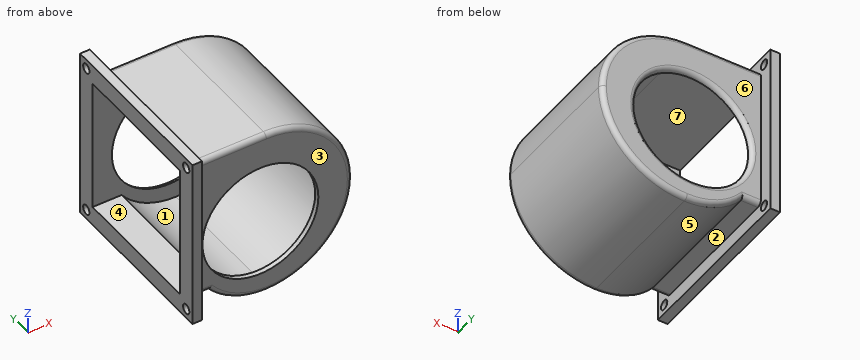
from build123d import *

# Parameters (mm, degrees)
PAD_DEPTH       = 28
THICKNESS_T     = 2
SKETCH001_R     = 24
POCKET_DEPTH    = 60.001
FILLET_R        = 1.9
SKETCH002_W     = 72
SKETCH002_H     = 72
SKETCH002_W_2   = 56
SKETCH002_H_2   = 56
PAD001_DEPTH    = 4
SKETCH003_R     = 2
POCKET001_DEPTH = 5


with BuildPart() as part:
    # Sketch → Pad (new body, symmetric)
    with BuildSketch(Plane.XZ):
        with BuildLine():
            Line((-32, -20), (-32, 36))
            Line((-32, 36), (2.5, 36))
            ThreePointArc((36, 2.5), (26.188077, 26.188077), (2.5, 36))
            ThreePointArc((2.5, -31), (26.188077, -21.188077), (36, 2.5))
            ThreePointArc((-19.994444, -20), (-10.019984, -28.102734), (2.5, -31))
            Line((-32, -20), (-19.994444, -20))
        make_face()
    extrude(amount=PAD_DEPTH, both=True)

    # Thickness
    thickness_openings = [part.faces().sort_by_distance(p)[0] for p in [
        (-32, 0, 8),
    ]]
    offset(amount=THICKNESS_T, openings=thickness_openings)

    # Sketch001 (on Face16 of Thickness) → Pocket (cut, through all)
    with BuildSketch(Plane.XZ.offset(30)):
        Circle(SKETCH001_R)
    extrude(amount=-POCKET_DEPTH, mode=Mode.SUBTRACT)

    # Fillet
    fillet_edges = [part.edges().sort_by_distance(p)[0] for p in [
        (-24, 30, 0),
    ]]
    fillet(fillet_edges, radius=FILLET_R)

    # Sketch002 (on Face3 of Fillet) → Pad001 (join)
    with BuildSketch(Plane(origin=(-32, 0, 0), x_dir=(0, -1, 0), z_dir=(-1, 0, 0))):
        with Locations((0, 8)):
            Rectangle(SKETCH002_W, SKETCH002_H)
        with Locations((0, 8)):
            Rectangle(SKETCH002_W_2, SKETCH002_H_2, mode=Mode.SUBTRACT)
    extrude(amount=-PAD001_DEPTH)

    # Sketch003 (on Face25 of Pad001) → Pocket001 (cut)
    with BuildSketch(Plane(origin=(-32, 0, 0), x_dir=(0, -1, 0), z_dir=(-1, 0, 0))):
        with Locations((-32, 40)):
            Circle(SKETCH003_R)
        with Locations((32, 40)):
            Circle(SKETCH003_R)
        with Locations((32, -24)):
            Circle(SKETCH003_R)
        with Locations((-32, -24)):
            Circle(SKETCH003_R)
    extrude(amount=-POCKET001_DEPTH, mode=Mode.SUBTRACT)


solid = part.part
Here's how the part is built. I have some questions about the finished solid (model axes, mm). Face numbers are marked on the shaded views. A direction names the side the tool comes from. Round coordinates to 2 decimals unless told otherwise and drop trailing zeros. Order: outer loops, then holes, each group sorted by start corner. A loop starts at its lowest first (then second) coordinate and runs counter-clockwise, first axis right, second up. Notation, with made-up numbers: (74.25, 6.25) -> (117.25, 6.25) arc R29 ccw to (117.25, 39.25) -> close; hole circle Ø11 at (73.25, 57.5). An arc over 180 degrees is marked (long way). Use CSV: the item, a comma, the result in double quotes.
1. I want a section at C-C on y = -16.5. List the corners of the cut face in (x, z) for me, and give its area (3 significant figures).
Recorded:
outline,"(-32, -28) -> (-28, -28) -> (-28, -22) -> (-20.95, -22) arc R30.5 ccw to (2.5, -33) arc R35.5 ccw to (38, 2.5) arc R35.5 ccw to (2.5, 38) -> (-28, 38) -> (-28, 44) -> (-32, 44) -> (-32, 36) -> (2.5, 36) arc R33.5 cw to (36, 2.5) arc R33.5 cw to (2.5, -31) arc R28.5 cw to (-19.99, -20) -> (-32, -20) -> close"
area,"409 mm2"
2. I need wall thicknesses on line 1 along Z through (x, y) = (-29.35, -32); line 2 along Z through (x, y) = (-26, -3); line 3 along X through (y, z) = (14.5, -24.5). Which ranges of each line are inside material? Lowest first, please.
Recorded:
line 1,"z = -28 to -26, -22 to 38, 42 to 44"
line 2,"z = -22 to -20, 36 to 38"
line 3,"x = -32 to -28, -18.62 to -15.62, 22.33 to 25.55"
3. I want a section at A-A on y = -32. List the corners of the cut face in (x, z) for me.
Recorded:
outline,"(-32, -28) -> (-28, -28) -> (-28, -26) -> (-32, -26) -> close; (-32, -22) -> (-28, -22) -> (-28, 38) -> (-32, 38) -> close; (-32, 42) -> (-28, 42) -> (-28, 44) -> (-32, 44) -> close"
4. I want a section at B-B on z = 40. List the corners of the cut face in (x, y) for me.
Recorded:
outline,"(-32, -36) -> (-28, -36) -> (-28, -34) -> (-32, -34) -> close; (-32, -30) -> (-28, -30) -> (-28, 30) -> (-32, 30) -> close; (-32, 34) -> (-28, 34) -> (-28, 36) -> (-32, 36) -> close"
5. I'm going to push flat-ended pins straight in: P1, Ø10, axis at x = -22.5, y = 20.5, coming from the -Z side; P2, Ø12, axis at y = 27.5, z = -17, coming from the -X side; P3, Ø3.5, axis at x = -25.5, y = 12.5, coming from the -Z side; P4, Ø5, axis at x = -0.5, z = 22, coming from the +Y side. Where does each tip first touch, or does it pass through?
Recorded:
P1,"stops at z = -25.53"
P2,"stops at x = -32"
P3,"stops at z = -22"
P4,"stops at y = 29.39"
6. Which directions (+Z, -Z, +X, -X, +Y, -Y) give clear straight access to the entire face, cutting with the end or side of a thin tool? Please do the marked faces 5, 6 and 7.
Recorded:
face 5,"-Z, +Y, -Y"
face 6,"+Z, -Z, +X, +Y"
face 7,"-X"
7. Thinking about a two-plate mould opening in Y: for the marked faces 1, 2, 3 and 4, which applies, pulls with the +Y half, pulls with the -Y half, needs draft (parallel to the pull), parting line crosses it, or undercut?
Recorded:
face 1,"undercut"
face 2,"needs draft"
face 3,"pulls with the -Y half"
face 4,"undercut"
8. I want a section at D-D on z = 0. Give the number of separate pieces and of enclosed holes in the cut face, and give its area (3 significant figures).
Recorded:
separate pieces,"3"
enclosed holes,"0"
area,"245 mm2"
